Part model, mm, in its own coordinate system. Face numbers are marked on the shaded views. A direction names the side the tool comes from. Round coordinates to 2 decimals unless told otherwise and drop trailing zeros. Write each loop counter-clockwise with the first axis right and the second up, starting at its lowest first coordinate (ties: lowest second). Pieces come first, ordered by that corner, then holes. Notation, with made-up numbers: M -39.5,89.25 L -30.5,89.25 A26 ccw -30.5,116.25 Z; hole C -34,28.5 d2. An arc over 180 degrees is marked long. Answer as a JSON object with one key per item and string values. Group by question number.
1. Drill centre lines: line 1 (X direction, y = 0, z = 10.75); line 2 (Z direction, x = -0.25, y = -5.25). Where is each one in solid material? Low to high. Write a range as from..to.
2. Band-saw the part on A-A, the plane z = 8.5. Write the cut outline in (x, y), plus the area to 3 significant figures.
3. Which spindle directions (+Z, -Z, +X, -X, +Y, -Y) get a long thin tool onto all of the face, cutting with end or side? Do the marked faces 1 and 2. Say none if no direction does.
4. Two-plate mould, pull along Y, no slides. Class the marked faces 3 and 4: +Y half, -Y half, draft (parallel to the pull), parting line (faces both ways), or undercut.
5. Drop flat-ended pins along their axis: pin 1 (4 mm diameter, centred on x = 2.5, y = -0.5, fed in from +Z); pin 2 (6 mm diameter, centred on x = -4, y = 5, fed in from -Z); pin 3 (5 mm diameter, centred on y = 5.5, z = 13, fed in from -X); pin 4 (5 mm diameter, centred on x = -5.5, z = 5.5, fed in from +Y). Give the stop position or say it passes through.
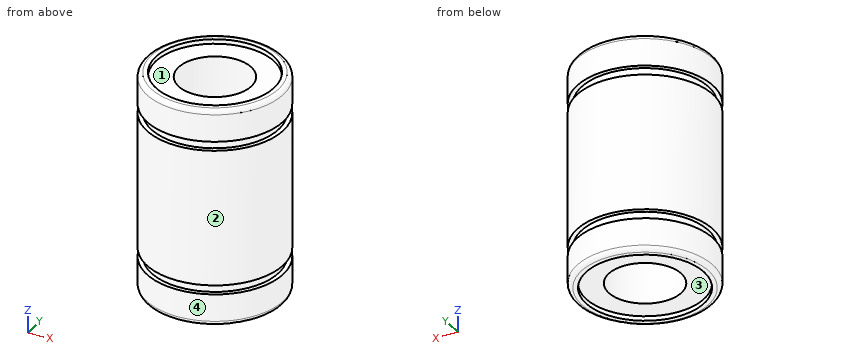
Autodesk Inventor part; units mm, degrees
ref_plane "YZ Plane" through (0, 0, 0) normal (1, 0, 0) x (0, 1, 0)
ref_plane "XZ Plane" through (0, 0, 0) normal (0, 1, 0) x (-1, 0, 0)
ref_plane "XY Plane" through (0, 0, 0) normal (0, 0, 1) x (1, 0, 0)
sketch "Sketch1" plane through (0, 0, 0) normal (0, 0, 1) x (1, 0, 0)
  circle A0 centre (0, 0) radius 4
  circle A1 centre (0, 0) radius 7.5
  dimension "d2" = 8
  dimension "d3" = 15
extrude "Extrusion1" add sketch "Sketch1" along normal blind 24
fillet "Fillet1" radius 0.5 2 edges at (-7.5, 0, 24) (-7.5, 0, 0)
sketch "Sketch2" plane through (0, 0, 0) normal (1, 0, 0) x (0, 1, 0)
  arc A0 (7, 0) -> (7.5, 0.5) centre (7, 0.5) ccw
  line L0 (7, 0) -> (4, 0)
  line L1 (4, 0) -> (4, 24)
  line L2 (4, 24) -> (7, 24)
  arc A1 (7.5, 23.5) -> (7, 24) centre (7, 23.5) ccw
  line L3 (7.5, 23.5) -> (7.5, 0.5)
  arc A2 (-7.5, 0.5) -> (-7, 0) centre (-7, 0.5) ccw
  line L4 (-7.5, 0.5) -> (-7.5, 23.5)
  arc A3 (-7, 24) -> (-7.5, 23.5) centre (-7, 23.5) ccw
  line L5 (-7, 24) -> (-4, 24)
  line L6 (-4, 24) -> (-4, 0)
  line L7 (-4, 0) -> (-7, 0)
  line L8 (7.5, 0.5) -> (7.5, 23.5)
  line L9 (7.5, 20.5) -> (7, 20.5)
  line L10 (7, 20.5) -> (7, 19.5)
  line L11 (7, 19.5) -> (7.5, 19.5)
  line L12 (7.5, 12) -> (4, 12) construction
  line L13 (7.5, 3.5) -> (7, 3.5)
  line L14 (7, 3.5) -> (7, 4.5)
  line L15 (7, 4.5) -> (7.5, 4.5)
  line L16 (-4, 24) -> (4, 24) construction
  line L17 (0, 24) -> (0, 0) construction
  point P0 (7.5, 3.5)
  point P1 (7.5, 4.5)
  dimension "d5" = 3.5
  dimension "d6" = 1
  dimension "d7" = 0.5
revolve "Revolution1" cut sketch "Sketch2" angle 360 about axis through (0, 0, 24) along (0, 0, -1) contours L13 L14 L15 L3 | L11 L10 L9 L3
sketch "Sketch3" plane through (0, 0, 24) normal (0, 0, 1) x (1, 0, 0)
  circle A0 centre (0, 0) radius 6.5
  circle A1 centre (0, 0) radius 7.5
  dimension "d9" = 1
extrude "Extrusion2" cut sketch "Sketch3" against normal blind 0.5 contours A0
extrude "Extrusion3" cut sketch "Sketch3" along normal blind 0.5 from surface at -24 contours A0
properties part number "berring" material "Aluminum 6061"
Worked answers:
{
 "1": {"line 1": "x = -7.5..-4, 4..7.5", "line 2": "z = 0.5..23.5"},
 "2": {"outline": "C 0,0 d15; hole C 0,0 d8", "area": "126 mm^2"},
 "3": {"face 1": "+Z", "face 2": "+Z, -Z"},
 "4": {"face 3": "undercut", "face 4": "parting line"},
 "5": {"pin 1": "stops at z = 23.5", "pin 2": "stops at z = 0", "pin 3": "stops at x = -6.87", "pin 4": "stops at y = 6.87"}
}
